Build history of the part. All positions in model axes, mm. A direction names the side the tool comes from. Round coordinates to 2 decimals unless told otherwise and drop trailing zeros. Write each loop counter-clockwise with the first axis right and the second up, starting at its lowest first coordinate (ties: lowest second). Pieces come first, ordered by that corner, then holes. Notation, with made-up numbers: M -39.75,-17 L -29.75,-17 A28 cw -29.75,13 Z; hole C 3,5 d8. An arc over 180 degrees is marked long. Write item = value, one per line.
from build123d import *

# Parameters (mm, degrees)
SALIENTE_EXTRUIR1_DEPTH = 18
SALIENTE_EXTRUIR2_START = 1.5
CROQUIS2_R              = 2.7
SALIENTE_EXTRUIR2_DEPTH = 1.5
SALIENTE_EXTRUIR3_DEPTH = 1.5
CROQUIS6_W              = 5.4
CROQUIS6_H              = 1.181933233
SALIENTE_EXTRUIR7_DEPTH = 10
CROQUIS7_W              = 5.4
CROQUIS7_H              = 10
CORTAR_EXTRUIR2_DEPTH   = 16.5
CROQUIS9_W              = 52.468080771
CROQUIS9_H              = 55.683263094
CORTAR_EXTRUIR3_DEPTH   = 30
CROQUIS10_W             = 2
CROQUIS10_H             = 3
CROQUIS10_H_2           = 2.995767736
CORTAR_EXTRUIR4_DEPTH   = 10
CROQUIS11_W             = 2.995767736
CROQUIS11_H             = 6.287117146
CROQUIS11_W_2           = 3
CROQUIS11_H_2           = 6.399149596
CORTAR_EXTRUIR5_DEPTH   = 7.4
CROQUIS12_W             = 3.7
CROQUIS12_H             = 3
REVOLUCI_N2_ANGLE       = 180


with BuildPart() as part:
    # Croquis1 → Saliente-Extruir1 (new body)
    with BuildSketch(Plane.XY):
        with BuildLine():
            Line((-54.535099114, 31.482780649), (-55.25791247, 32.775048384))
            Line((-55.25791247, 32.775048384), (-58.679569293, 30.903614553))
            ThreePointArc((-58.679569293, 30.903614553), (-72.555259572, 38.768368337), (-85.712228427, 29.752642999))
            Line((-85.712228427, 29.752642999), (-86.469958437, 28.480534403))
            Line((-86.469958437, 28.480534403), (-83.138420786, 26.453009587))
            ThreePointArc((-83.138420786, 26.453009587), (-83.011652218, 10.503932418), (-68.625320614, 3.617525822))
            Line((-68.625320614, 3.617525822), (-67.144777249, 3.597366682))
            Line((-67.144777249, 3.597366682), (-67.054658077, 7.49632533))
            ThreePointArc((-67.054658077, 7.49632533), (-53.305736365, 15.580648714), (-54.535099114, 31.482780649))
        make_face()
        with BuildLine():
            Line((-69.624216052, 5.117649823), (-68.624216052, 5.117649823))
            Line((-68.624216052, 5.117649823), (-68.624216052, 9.117649823))
            ThreePointArc((-68.624216052, 9.117649823), (-55.305921191, 15.218525867), (-55.334796889, 29.867649823))
            Line((-55.334796889, 29.867649823), (-55.834796889, 30.733675227))
            Line((-55.834796889, 30.733675227), (-59.298898504, 28.733675227))
            ThreePointArc((-59.298898504, 28.733675227), (-71.241559574, 37.21721889), (-83.913635214, 29.867649823))
            Line((-83.913635214, 29.867649823), (-84.413635214, 29.001624419))
            Line((-84.413635214, 29.001624419), (-80.949533599, 27.001624419))
            ThreePointArc((-80.949533599, 27.001624419), (-82.325167391, 12.417204713), (-69.624216052, 5.117649823))
        make_face(mode=Mode.SUBTRACT)
    extrude(amount=SALIENTE_EXTRUIR1_DEPTH)

    # Croquis2 → Saliente-Extruir2 (add)
    with BuildSketch(Plane(origin=(0, 0, 0), x_dir=(-1, 0, 0), z_dir=(0, 0, -1)).offset(SALIENTE_EXTRUIR2_START)):
        with BuildLine():
            Line((67.054658077, 7.49632533), (67.144777249, 3.597366682))
            Line((67.144777249, 3.597366682), (68.625320614, 3.617525822))
            ThreePointArc((68.625320614, 3.617525822), (83.011652218, 10.503932418), (83.138420786, 26.453009587))
            Line((83.138420786, 26.453009587), (86.469958437, 28.480534403))
            Line((86.469958437, 28.480534403), (85.712228427, 29.752642999))
            ThreePointArc((85.712228427, 29.752642999), (72.555259572, 38.768368337), (58.679569293, 30.903614553))
            Line((58.679569293, 30.903614553), (55.25791247, 32.775048384))
            Line((55.25791247, 32.775048384), (54.535099114, 31.482780649))
            ThreePointArc((54.535099114, 31.482780649), (53.305736365, 15.580648714), (67.054658077, 7.49632533))
        make_face()
        with Locations((69.624216052, 21.617649823)):
            Circle(CROQUIS2_R, mode=Mode.SUBTRACT)
    extrude(amount=-SALIENTE_EXTRUIR2_DEPTH)

    # Croquis3 → Saliente-Extruir3 (add)
    with BuildSketch(Plane.XY.offset(18)):
        with BuildLine():
            Line((-67.144777249, 3.597366682), (-67.054658077, 7.49632533))
            ThreePointArc((-67.054658077, 7.49632533), (-53.305736365, 15.580648714), (-54.535099114, 31.482780649))
            Line((-54.535099114, 31.482780649), (-55.25791247, 32.775048384))
            Line((-55.25791247, 32.775048384), (-58.679569293, 30.903614553))
            ThreePointArc((-58.679569293, 30.903614553), (-72.555259572, 38.768368337), (-85.712228427, 29.752642999))
            Line((-85.712228427, 29.752642999), (-86.469958437, 28.480534403))
            Line((-86.469958437, 28.480534403), (-83.138420786, 26.453009587))
            ThreePointArc((-83.138420786, 26.453009587), (-83.011652218, 10.503932418), (-68.625320614, 3.617525822))
            Line((-68.625320614, 3.617525822), (-67.144777249, 3.597366682))
        make_face()
    extrude(amount=SALIENTE_EXTRUIR3_DEPTH)

    # Croquis6 → Saliente-Extruir7 (add)
    with BuildSketch(Plane(origin=(0, 0, -1.5), x_dir=(-1, 0, 0), z_dir=(0, 0, -1))):
        with Locations((69.624216052, 21.026683207)):
            Rectangle(CROQUIS6_W, CROQUIS6_H)
    extrude(amount=SALIENTE_EXTRUIR7_DEPTH)

    # Croquis7 → Cortar-Extruir2 (cut)
    with BuildSketch(Plane(origin=(0, 21.617649823, 0), x_dir=(1, 0, 0), z_dir=(0, 1, 0))):
        with Locations((-69.624216052, 6.5)):
            Rectangle(CROQUIS7_W, CROQUIS7_H)
    extrude(amount=-CORTAR_EXTRUIR2_DEPTH, mode=Mode.SUBTRACT)

    # Croquis8 → Revolución1 (revolve)
    with BuildSketch(Plane(origin=(0, 21.617649823, 0), x_dir=(1, 0, 0), z_dir=(0, 1, 0)), mode=Mode.PRIVATE) as revoluci_n1_sk:
        Polygon((-72.324216052, 1.5), (-79.486781688, 1.5), (-72.324216052, 11.5), align=None)
        Polygon((-72.324216052, -19.5), (-69.624216052, -19.5), (-69.624216052, -25.5), (-72.324216052, -25.5), (-77.324216052, -25.5), (-77.324216052, -19.5), align=None)
    revolve(revoluci_n1_sk.sketch.rotate(Axis((-69.624216052, 21.617649823, 19.5), (0, 0, 1)), 180), axis=Axis((-69.624216052, 21.617649823, 19.5), (0, 0, 1)))

    # Croquis9 → Cortar-Extruir3 (cut)
    with BuildSketch(Plane(origin=(0, 21.617649823, 0), x_dir=(1, 0, 0), z_dir=(0, 1, 0))):
        with Locations((-61.70964897, -8.735329994)):
            Rectangle(CROQUIS9_W, CROQUIS9_H)
    extrude(amount=-CORTAR_EXTRUIR3_DEPTH, mode=Mode.SUBTRACT)

    # Croquis10 → Cortar-Extruir4 (cut)
    with BuildSketch(Plane.XZ.offset(-21.617649823)):
        with Locations((-64.924216052, -4)):
            Rectangle(CROQUIS10_W, CROQUIS10_H)
        with Locations((-74.324216052, -4)):
            Rectangle(CROQUIS10_W, CROQUIS10_H)
        with Locations((-64.924216052, 22.347883868)):
            Rectangle(CROQUIS10_W, CROQUIS10_H_2)
        with Locations((-74.324216052, 22.347883868)):
            Rectangle(CROQUIS10_W, CROQUIS10_H_2)
    extrude(amount=-CORTAR_EXTRUIR4_DEPTH, mode=Mode.SUBTRACT)

    # Croquis11 → Cortar-Extruir5 (cut)
    with BuildSketch(Plane.ZY.offset(73.324216052)):
        with Locations((22.347883868, 29.264688265)):
            Rectangle(CROQUIS11_W, CROQUIS11_H)
        with Locations((-4, 30.385140174)):
            Rectangle(CROQUIS11_W_2, CROQUIS11_H_2)
    extrude(amount=-CORTAR_EXTRUIR5_DEPTH, mode=Mode.SUBTRACT)

    # Croquis12 → Revolución2 (revolve)
    with BuildSketch(Plane.XZ.offset(-21.617649823)):
        with Locations((-71.474216052, 16.5)):
            Rectangle(CROQUIS12_W, CROQUIS12_H)
    revolve(axis=Axis((-69.624216052, 21.617649823, 18), (0, 0, -1)), revolution_arc=REVOLUCI_N2_ANGLE)


solid = part.part
1. Band-saw the part on A-A (y = 34.5). List the corners of the cut face in (x, z), plus the area to 3 significant figures.
Responses:
outline = M -82.43,-1.5 L -61.4,-1.5 L -61.4,19.5 L -82.43,19.5 Z; hole M -80.02,0 L -63.71,0 L -63.71,18 L -80.02,18 Z
area = 148 mm²
2. Probe probe 1 along Z at (x, y) = (-79, 26.5); probe 2 along X at (y, z) = (23.5, 21); probe 3 along X at (y, z) = (25, 16). List the from-to ranges inside material, lowest first.
Responses:
probe_1 = -1.5 to 0, 18 to 19.5
probe_2 = -77.09 to -75.32, -73.32 to -65.92, -63.92 to -62.16
probe_3 = -83.92 to -82.25, -71.12 to -68.12, -53.4 to -51.8
3. Tool access for faces 1 (the face through (-84.828, 27.481, 8.853)), 2 (the face through (-70, 23, 15)), 3 (the face through (-69.455, 29.316, 24.458)): list every direction of +Z, -Z, +X, -X, +Y, -Y with a clear straight run to the whole face (end or side of a thin tool).
Responses:
face_1 = +Z, -Z, -X
face_2 = -Y
face_3 = +Z, +Y
4. Band-saw the part on D-D (z = -3.5). List the corners of the cut face in (x, y).
Responses:
outline = M -78.05,21.62 L -75.32,21.62 L -75.32,27.83 A8.43 ccw Z; M -73.32,21.62 L -72.32,21.62 A2.7 cw -66.92,21.62 L -65.92,21.62 L -65.92,27.19 L -73.32,27.19 Z; M -63.92,21.62 L -61.19,21.62 A8.43 ccw -63.92,27.83 Z
5. Band-saw the part on B-B (x = -81.5). List the corners of the cut face in (y, z), plus the area to 3 significant figures.
Responses:
outline = M 21.62,-1.5 L 35.34,-1.5 L 35.34,19.5 L 21.62,19.5 L 21.62,18 L 26.25,18 L 26.25,0 L 21.62,0 Z; hole M 27.32,0 L 33.2,0 L 33.2,18 L 27.32,18 Z
area = 98.8 mm²
6. Mould opens along Z. For faces 4 (the face through (-70, 28, -2.5)), 5 (the face through (-54.89, 32.12, 8.85)), 6 (the face through (-69, 32, -1.5)) say: pulls with the +Z half, pulls with the -Z half, needs draft (parallel to the pull), parting line crosses it, or undercut.
Responses:
face_4 = undercut
face_5 = needs draft
face_6 = pulls with the -Z half
7. Flat gauge pins, fed straight in: pin 1 (5 mm diameter, centred on x = -68, y = 28.5, fed in from -Z); pin 2 (10 mm diameter, centred on x = -65, y = 32.5, fed in from +Z); pin 3 (1 mm diameter, centred on x = -78.5, z = 8.5, fed in from -Y); pin 4 (1.5 mm diameter, centred on x = -69, z = 22, fed in from +Y). Where does each tip first touch, or does it go through?
Responses:
pin_1 = -8.89
pin_2 = 25.5
pin_3 = 35.2
pin_4 = 26.12
8. Band-saw the part on C-C (z = 15.5). List the corners of the cut face in (x, y), plus the area to 3 significant figures.
Responses:
outline = M -86.47,28.48 L -83.14,26.45 A15.06 ccw -85.05,21.62 L -83.51,21.62 A13.54 cw -80.95,27 L -84.41,29 L -83.91,29.87 A13.54 cw -59.3,28.73 L -55.83,30.73 L -55.33,29.87 A13.54 cw -53.2,21.62 L -51.63,21.62 A15.06 ccw -54.54,31.48 L -55.26,32.78 L -58.68,30.9 A15.06 ccw -85.71,29.75 Z; M -73.32,21.62 L -65.92,21.62 A3.7 ccw Z
area = 111 mm²
